```python
from build123d import *

# Parameters (mm, degrees)
SKETCH5_OUTSIDE_W   = 34.468
SKETCH5_OUTSIDE_H   = 34.468
CUT_EXTRUDE1_DEPTH  = 7.2
BOSS_EXTRUDE1_REACH = 51.718
SKETCH10_R          = 10.705
SKETCH10_R_2        = 6.9
BOSS_EXTRUDE3_REACH = 31.655
SKETCH12_R          = 8.3
CUT_EXTRUDE3_REACH  = 53.775
SKETCH13_R          = 3.45
SKETCH14_R          = 23.979548074
CUT_EXTRUDE5_DEPTH  = 32
BOSS_EXTRUDE4_START = 2
SKETCH16_R          = 30.1625
SKETCH16_R_2        = 7.874
BOSS_EXTRUDE4_DEPTH = 2
BOSS_EXTRUDE5_START = 80
SKETCH17_R          = 30.1625
SKETCH17_R_2        = 25.4
BOSS_EXTRUDE5_DEPTH = 80
SKETCH18_R          = 1.7
BOSS_EXTRUDE6_DEPTH = 2


# Read off the part's stored shape, not the designer's step: Cut-Extrude2
with BuildPart() as part:
    # Sketch1 → Revolve1 (revolve)
    with BuildSketch(Plane.XY, mode=Mode.PRIVATE) as revolve1_sk:
        Polygon((3.25, 47.7), (4.8, 47.7), (5.2, 43.217813034), (4.8, 42.533333333), (5.2, 38.051146367), (4.8, 37.366666667), (5.2, 32.8844797), (4.8, 32.2), (5.25, 26.2), (5.25, 22.2), (10.6, 22.2), (10.6, 15), (8.3, 15), (8.3, 0), (5.5, 0), (5.5, 18), (3.25, 19.7), align=None)
    revolve(revolve1_sk.sketch.rotate(Axis((0, 0, 0), (0, 1, 0)), 90), axis=Axis((0, 0, 0), (0, 1, 0)))

    # Sketch5 outside → Cut-Extrude1 (cut)
    with BuildSketch(Plane(origin=(0, 22.2, 0), x_dir=(1, 0, 0), z_dir=(0, 1, 0))):
        Rectangle(SKETCH5_OUTSIDE_W, SKETCH5_OUTSIDE_H)
        Polygon((-5.3, 9.17986928), (5.3, 9.17986928), (10.6, 0), (5.3, -9.17986928), (-5.3, -9.17986928), (-10.6, 0), align=None, mode=Mode.SUBTRACT)
    extrude(amount=-CUT_EXTRUDE1_DEPTH, mode=Mode.SUBTRACT)

    # Sketch4 → Cut-Revolve1 (revolve, cut)
    with BuildSketch(Plane.XY, mode=Mode.PRIVATE) as cut_revolve1_sk:
        Polygon((6.9, 0), (8.3, 1.4), (8.3, 0), align=None)
        Polygon((8.3, 15), (10.6, 15.837131539), (10.6, 15), align=None)
        Polygon((8.3, 22.2), (10.6, 21.362868461), (10.6, 22.2), align=None)
    revolve(cut_revolve1_sk.sketch.rotate(Axis((0, 0, 0), (0, 1, 0)), 90), axis=Axis((0, 0, 0), (0, 1, 0)), mode=Mode.SUBTRACT)

    # Boss-Extrude1: up to this cone (the profile starts outside it)
    boss_extrude1_end = Plane(origin=(0, 0, 0), z_dir=(0, 1, 0)).offset(11.979048056) * Cone(2.747e-06, 110.555614597, 40.238951944, align=(Align.CENTER, Align.CENTER, Align.MIN), mode=Mode.PRIVATE)
    # Sketch10 → Boss-Extrude1 (add, up to the surface)
    with BuildSketch(Plane.XZ, mode=Mode.PRIVATE) as boss_extrude1_sk1:
        with Locations(Location((0, 0, 0), (0, 0, 270))):
            Circle(SKETCH10_R)
        Circle(SKETCH10_R_2, mode=Mode.SUBTRACT)
    boss_extrude1_tool1 = extrude(boss_extrude1_sk1.sketch, amount=-BOSS_EXTRUDE1_REACH, mode=Mode.PRIVATE) - boss_extrude1_end
    add(boss_extrude1_tool1.solids().sort_by_distance((0, 0, 10.402217))[0])

    # Cut-Extrude2 outline → Cut-Extrude2 (revolve, cut)
    with BuildSketch(Plane.XY):
        Polygon((7.874, 16.206311111), (5.5, 18), (5.5, 0), (7.874, 0), align=None)
    revolve(axis=Axis((0, 0, 0), (0, 1, 0)), mode=Mode.SUBTRACT)

    # Boss-Extrude3: up to this cone (the profile starts inside it)
    boss_extrude3_end = Plane(origin=(0, 22.2, 0), z_dir=(0, 1, 0)).offset(-10.220951944) * Cone(2.747e-06, 193.581188051, 70.457789364, align=(Align.CENTER, Align.CENTER, Align.MIN), mode=Mode.PRIVATE)
    # Sketch12 → Boss-Extrude3 (add, up to the surface)
    with BuildSketch(Plane(origin=(0, 22.2, 0), x_dir=(1, 0, 0), z_dir=(0, 1, 0)), mode=Mode.PRIVATE) as boss_extrude3_sk1:
        Polygon((-7.609401077, 13.17986928), (-15.218802154, 0), (-7.609401077, -13.17986928), (7.609401077, -13.17986928), (15.218802154, 0), (7.609401077, 13.17986928), align=None)
        Circle(SKETCH12_R, mode=Mode.SUBTRACT)
    boss_extrude3_tool1 = extrude(boss_extrude3_sk1.sketch, amount=-BOSS_EXTRUDE3_REACH, mode=Mode.PRIVATE) & boss_extrude3_end
    add(boss_extrude3_tool1.solids().sort_by_distance((-11.065395, 22.2, -6.388609))[0])

    # Cut-Extrude3: up to this cone (the profile starts outside it)
    cut_extrude3_end = Plane(origin=(0, 47.7, 0), z_dir=(0, -1, 0)).offset(25.544445444) * Cone(1.324e-06, 38.025735294, 28.730554556, align=(Align.CENTER, Align.CENTER, Align.MIN), mode=Mode.PRIVATE)
    # Sketch13 → Cut-Extrude3 (cut, up to the surface)
    with BuildSketch(Plane(origin=(0, 47.7, 0), x_dir=(1, 0, 0), z_dir=(0, 1, 0)), mode=Mode.PRIVATE) as cut_extrude3_sk1:
        with Locations(Location((0, 0, 0), (0, 0, 270))):
            Circle(SKETCH13_R)
    cut_extrude3_tool1 = extrude(cut_extrude3_sk1.sketch, amount=-CUT_EXTRUDE3_REACH, mode=Mode.PRIVATE) - cut_extrude3_end
    add(cut_extrude3_tool1.solids().sort_by_distance((0, 47.7, 0))[0], mode=Mode.SUBTRACT)

    # Sketch14 → Cut-Extrude5 (cut)
    with BuildSketch(Plane(origin=(0, 47.7, 0), x_dir=(1, 0, 0), z_dir=(0, 1, 0))):
        Circle(SKETCH14_R)
    extrude(amount=-CUT_EXTRUDE5_DEPTH, mode=Mode.SUBTRACT)

    # Sketch16 → Boss-Extrude4 (add)
    with BuildSketch(Plane(origin=(0, 15.7, 0), x_dir=(1, 0, 0), z_dir=(0, 1, 0)).offset(BOSS_EXTRUDE4_START)):
        with Locations(Location((0, 0, 0), (0, 0, 270))):
            Circle(SKETCH16_R)
        with Locations(Location((0, 0, 0), (0, 0, 90))):
            Circle(SKETCH16_R_2, mode=Mode.SUBTRACT)
    extrude(amount=-BOSS_EXTRUDE4_DEPTH)

    # Sketch17 → Boss-Extrude5 (add)
    with BuildSketch(Plane(origin=(0, 17.7, 0), x_dir=(1, 0, 0), z_dir=(0, 1, 0)).offset(BOSS_EXTRUDE5_START)):
        with Locations(Location((0, 0, 0), (0, 0, 270))):
            Circle(SKETCH17_R)
        with Locations(Location((0, 0, 0), (0, 0, 270))):
            Circle(SKETCH17_R_2, mode=Mode.SUBTRACT)
    extrude(amount=-BOSS_EXTRUDE5_DEPTH)

    # Sketch18 → Boss-Extrude6 (add)
    # profile 1 of 8: a face of its own
    with BuildSketch(Plane(origin=(0, 97.7, 0), x_dir=(1, 0, 0), z_dir=(0, 1, 0))):
        with BuildLine():
            ThreePointArc((-29.745191313, -5), (-30.1625, 0), (-29.745191313, 5))
            Line((-29.745191313, 5), (-41.745191313, 5))
            Line((-41.745191313, 5), (-41.745191313, -5))
            Line((-41.745191313, -5), (-29.745191313, -5))
        make_face()
        with Locations(Location((-36.745191313, 0, 0), (0, 0, 270))):
            Circle(SKETCH18_R, mode=Mode.SUBTRACT)
    # profile 2 of 8: a face of its own
    with BuildSketch(Plane(origin=(0, 97.7, 0), x_dir=(1, 0, 0), z_dir=(0, 1, 0))):
        with BuildLine():
            Line((-29.745191313, -5), (-29.745191313, 5))
            ThreePointArc((-29.745191313, 5), (-30.1625, 0), (-29.745191313, -5))
        make_face()
    # profile 3 of 8: a face of its own
    with BuildSketch(Plane(origin=(0, 97.7, 0), x_dir=(1, 0, 0), z_dir=(0, 1, 0))):
        with BuildLine():
            ThreePointArc((29.745191313, -5), (30.1625, 0), (29.745191313, 5))
            Line((29.745191313, 5), (29.745191313, -5))
        make_face()
    # profile 4 of 8: a face of its own
    with BuildSketch(Plane(origin=(0, 97.7, 0), x_dir=(1, 0, 0), z_dir=(0, 1, 0))):
        with BuildLine():
            Line((41.745191313, 5), (29.745191313, 5))
            ThreePointArc((29.745191313, 5), (30.1625, 0), (29.745191313, -5))
            Line((29.745191313, -5), (41.745191313, -5))
            Line((41.745191313, -5), (41.745191313, 5))
        make_face()
        with Locations(Location((36.745191313, 0, 0), (0, 0, 270))):
            Circle(SKETCH18_R, mode=Mode.SUBTRACT)
    # profile 5 of 8: a face of its own
    with BuildSketch(Plane(origin=(0, 97.7, 0), x_dir=(1, 0, 0), z_dir=(0, 1, 0))):
        with BuildLine():
            ThreePointArc((5, -29.745191313), (0, -30.1625), (-5, -29.745191313))
            Line((-5, -29.745191313), (-5, -41.745191313))
            Line((-5, -41.745191313), (5, -41.745191313))
            Line((5, -41.745191313), (5, -29.745191313))
        make_face()
        with Locations(Location((0, -36.745191313, 0), (0, 0, 270))):
            Circle(SKETCH18_R, mode=Mode.SUBTRACT)
    # profile 6 of 8: a face of its own
    with BuildSketch(Plane(origin=(0, 97.7, 0), x_dir=(1, 0, 0), z_dir=(0, 1, 0))):
        with BuildLine():
            Line((5, -29.745191313), (-5, -29.745191313))
            ThreePointArc((-5, -29.745191313), (0, -30.1625), (5, -29.745191313))
        make_face()
    # profile 7 of 8: a face of its own
    with BuildSketch(Plane(origin=(0, 97.7, 0), x_dir=(1, 0, 0), z_dir=(0, 1, 0))):
        with BuildLine():
            ThreePointArc((5, 29.745191313), (0, 30.1625), (-5, 29.745191313))
            Line((-5, 29.745191313), (5, 29.745191313))
        make_face()
    # profile 8 of 8: a face of its own
    with BuildSketch(Plane(origin=(0, 97.7, 0), x_dir=(1, 0, 0), z_dir=(0, 1, 0))):
        with BuildLine():
            Line((-5, 41.745191313), (-5, 29.745191313))
            ThreePointArc((-5, 29.745191313), (0, 30.1625), (5, 29.745191313))
            Line((5, 29.745191313), (5, 41.745191313))
            Line((5, 41.745191313), (-5, 41.745191313))
        make_face()
        with Locations(Location((0, 36.745191313, 0), (0, 0, 270))):
            Circle(SKETCH18_R, mode=Mode.SUBTRACT)
    extrude(amount=-BOSS_EXTRUDE6_DEPTH)


solid = part.part
```
Verification items for the finished model (mm, model axes). A direction names the side the tool comes from. Round coordinates to 2 decimals unless told otherwise and drop trailing zeros. Order: outer loops, then holes, each group sorted by start corner. A loop starts at its lowest first (then second) coordinate and runs counter-clockwise, first axis right, second up. Notation, with made-up numbers: (60.5, 40) - (107.5, 40) arc R18 ccw to (107.5, 58) - close; hole circle Ø9 at (-35, 76.5). An arc over 180 degrees is marked (long way). Use CSV: the item, a comma, the result in double quotes. Start each with the question number.
1) Section check C-C, the plane y = 90. Record the cut outline in (x, z) (1 decimal).
2) Access from +Z, -Z, +X, -X, +Y, -Y to the whole of each face (thin tool, end or side, straight path). Record for faces 1 (the flat face through (0, 15.7, 13)), 2 (the flat face through (6, 17.7, -6)), 3 (the flat face through (6, 0, 6)).
3) Section check D-D, the plane y = 10.5. Record the cut outline in (x, z) (3 decimals).
4) Thickness scan on L1, parallel to X at y = 97, z = 0; L2, parallel to X at y = 35, z = 0; L3, parallel to Z at x = -3, y = 27. Record the ranges inside material, lowest first.
5) Go/stop test with flat-tipped pins: P1, Ø1.6, axis at y = 96.5, z = 34, coming from the -X side; P2, Ø8, axis at x = 7, z = 29, coming from the -Y side; P3, Ø1.5, axis at y = 51.5, z = -4.5, coming from the +X side; P4, Ø9.5, axis at x = 0, z = 0, coming from the -Y side. Record where each tip stops, or that it passes through.
6) Section check A-A, the plane z = -19.5. Record the cut outline in (x, y).
7) Mould release check, pull along X, two halves, no side actions. Record for faces 4 (the flat face through (-34, 95.7, 0)), 5 (the cylindrical face through (9.06, 57.27, 28.77)), 6 (the cylindrical face through (-35.596, 96.714, -1.253)), 7 (the cylindrical face through (-15.456, 58.26, -20.157)): +X half, -X half, draft (parallel to the pull), parting line (faces both ways), or undercut.
8) Section check B-B, the plane x = -15. Record the cut outline in (y, z).
Answers:
1,outline,"circle Ø60.3 at (0, 0); hole circle Ø50.8 at (0, 0)"
2,face 1,"-Y"
2,face 2,"+Y"
2,face 3,"+Z, -Z, +X, -X, -Y"
3,outline,"circle Ø21.41 at (0, 0); hole circle Ø15.748 at (0, 0)"
4,L1,"x = -41.75 to -38.45, -35.05 to -25.4, 25.4 to 35.05, 38.45 to 41.75"
4,L2,"x = -30.16 to -25.4, 25.4 to 30.16"
4,L3,"z = -30.01 to -25.22, 25.22 to 30.01"
5,P1,"stops at x = -5"
5,P2,"stops at y = 15.7"
5,P3,"stops at x = 29.93"
5,P4,"passes through"
6,outline,"(-23.01, 15.7) - (23.01, 15.7) - (23.01, 97.7) - (16.28, 97.7) - (16.28, 17.7) - (-16.28, 17.7) - (-16.28, 97.7) - (-23.01, 97.7) - close"
7,face 4,"draft"
7,face 5,"parting line"
7,face 6,"undercut"
7,face 7,"undercut"
8,outline,"(15.7, -26.17) - (97.7, -26.17) - (97.7, -20.5) - (17.7, -20.5) - (17.7, 20.5) - (97.7, 20.5) - (97.7, 26.17) - (15.7, 26.17) - close"
